```python
from build123d import *

# Parameters (mm, degrees)
BOSS_EXTRUDE1_DEPTH = 12.7
FILLET1_R           = 6.35
SKETCH2_R           = 3.81
CUT_EXTRUDE1_DEPTH  = 310.525863217
SKETCH3_R           = 3.81
CUT_EXTRUDE2_DEPTH  = 310.525863217


with BuildPart() as part:
    # Sketch1 → Boss-Extrude1 (new body)
    with BuildSketch(Plane(origin=(0, 0, 0), x_dir=(1, 0, 0), z_dir=(0, 1, 0))):
        with BuildLine():
            Line((0, 0), (12.7, 0))
            Line((12.7, 0), (12.7, -50.8))
            ThreePointArc((12.7, -50.8), (23.859231637, -77.740768363), (50.8, -88.9))
            ThreePointArc((50.8, -88.9), (77.740768363, -77.740768363), (88.9, -50.8))
            Line((88.9, -50.8), (88.9, 0))
            Line((88.9, 0), (101.6, 0))
            Line((101.6, 0), (101.6, -76.2))
            ThreePointArc((101.6, -76.2), (74.907118974, -158.75), (101.6, -241.3))
            Line((101.6, -241.3), (101.6, -292.1))
            Line((101.6, -292.1), (88.9, -292.1))
            Line((88.9, -292.1), (88.9, -266.7))
            ThreePointArc((88.9, -266.7), (77.740768363, -239.759231637), (50.8, -228.6))
            ThreePointArc((50.8, -228.6), (23.859231637, -239.759231637), (12.7, -266.7))
            Line((12.7, -266.7), (12.7, -292.1))
            Line((12.7, -292.1), (0, -292.1))
            Line((0, -292.1), (0, -241.3))
            ThreePointArc((0, -241.3), (26.692881026, -158.75), (0, -76.2))
            Line((0, -76.2), (0, 0))
        make_face()
    extrude(amount=BOSS_EXTRUDE1_DEPTH)

    # Fillet1
    fillet1_edges = [part.edges().sort_by_distance(p)[0] for p in [
        (95.25, 0, 0),
        (6.35, 0, 0),
        (95.25, 12.7, 0),
        (6.35, 12.7, 0),
        (6.35, 0, 292.1),
        (6.35, 12.7, 292.1),
        (95.25, 0, 292.1),
        (95.25, 12.7, 292.1),
    ]]
    fillet(fillet1_edges, radius=FILLET1_R - 0.0001)  # a hair under: the kernel refuses the full size

    # Sketch2 → Cut-Extrude1 (cut, through all)
    with BuildSketch(Plane(origin=(101.6, 0, 0), x_dir=(0, 0, -1), z_dir=(1, 0, 0))):
        with Locations((-285.75, 6.35)):
            Circle(SKETCH2_R)
    extrude(amount=-CUT_EXTRUDE1_DEPTH, mode=Mode.SUBTRACT)

    # Sketch3 → Cut-Extrude2 (cut, through all)
    with BuildSketch(Plane(origin=(101.6, 0, 0), x_dir=(0, 0, -1), z_dir=(1, 0, 0))):
        with Locations((-6.35, 6.35)):
            Circle(SKETCH3_R)
    extrude(amount=-CUT_EXTRUDE2_DEPTH, mode=Mode.SUBTRACT)


solid = part.part
```
Input: part model. Units: mm. Frame: model coordinates. A direction names the side the tool comes from. Round coordinates to 2 decimals unless told otherwise and drop trailing zeros. Order: outer loops, then holes, each group sorted by start corner. A loop starts at its lowest first (then second) coordinate and runs counter-clockwise, first axis right, second up. Notation, with made-up numbers: (45.25, 31) - (89.25, 31) arc R20 cw to (89.25, 64) - close; hole circle Ø10 at (-14, 58). An arc over 180 degrees is marked (long way). One line per question, with ' | ' between items. Start each with the question number.
1) Cut plane B-B, the plane z = 58.5. Return the cut outline in (x, y), then the cut area to 3 significant figures.
2) Set-up query: faces 1 (the cylindrical face through (95.16, 10.79, 290.29)), 2 (the flat face through (12.7, 6, 276)). Return all of +Z, -Z, +X, -X, +Y, -Y with unobstructed straight access to the full face (end or side cutting, diameter ignored); none if empty.
3) Pull-direction query (Z, two-part tool) for faces 3 (the cylindrical face through (6.439, 6.518, 289.556)), 4 (the cylindrical face through (95.339, 6.518, 289.556)), 5 (the cylindrical face through (95.34, 10.79, 1.81)), 6 (the flat face through (88.9, 6, 26)); classes: +Z half, -Z half, draft (parallel to the pull), parting line (faces both ways), or undercut.
4) Contact query for flat-ended pins moving along their axis: P1, Ø6.5, axis at y = 3.5, z = 38, coming from the -X side; P2, Ø6, axis at x = 61, y = 2, coming from the -Z side; P3, Ø5, axis at y = 5, z = 216, coming from the +X side; P4, Ø4.5, axis at y = 6.35, z = 6.35, coming from the -X side. Output: stop coordinate, or through.
5) Cut plane C-C, the plane x = 42.5. Return the cut outline in (y, z).
6) Cut plane D-D, the plane z = 222. Return the cut outline in (x, y).
7) Ray query, probe 1 along Z at (x, y) = (6.5, 7); probe 2 along Z at (x, y) = (90, 6.5); probe 3 along Y at (x, z) = (4, 285.75). Return the intervals inside material, ascending.
8) Cut plane A-A, the plane x = 7.5. Give the number of separate pieces and of enclosed holes in the cut face, then the cut area to 3 significant figures.
Worked out:
1) outline: (0, 0) - (13.49, 0) - (13.49, 12.7) - (0, 12.7) - close; (88.11, 0) - (101.6, 0) - (101.6, 12.7) - (88.11, 12.7) - close | area: 343 mm^2
2) face 1: +Z, +X, -X, +Y | face 2: +Z, +Y, -Y
3) face 3: undercut | face 4: undercut | face 5: -Z half | face 6: draft
4) P1: stops at x = 0 | P2: stops at z = 86.54 | P3: stops at x = 88.19 | P4: passes through
5) outline: (0, 87.98) - (12.7, 87.98) - (12.7, 229.52) - (0, 229.52) - close
6) outline: (11.71, 0) - (89.89, 0) - (89.89, 12.7) - (11.71, 12.7) - close
7) probe 1: z = 0.03 to 2.6, 10.1 to 86.04, 231.46 to 282, 289.5 to 292.07 | probe 2: z = 0 to 2.54, 10.16 to 95.28, 222.22 to 281.94, 289.56 to 292.1 | probe 3: y = 0 to 2.54, 10.16 to 12.7
8) separate pieces: 2 | enclosed holes: 2 | area: 1,780 mm^2
